Autodesk Inventor part; units mm, degrees
ref_plane "YZ Plane" through (0, 0, 0) normal (1, 0, 0) x (0, 1, 0)
ref_plane "XY Plane" through (0, 0, 0) normal (0, 0, 1) x (1, 0, 0)
sketch "Sketch1" plane through (0, 0, 0) normal (0, 1, 0) x (-1, 0, 0)
  line L0 (20, 0) -> (0, 0)
  line L1 (0, 0) -> (0, -41)
  line L2 (0, -41) -> (20, -41)
  line L3 (20, -41) -> (20, 0)
  dimension "d0" = 20
  dimension "d1" = 41
extrude "Extrusion1" add sketch "Sketch1" along normal blind 37.5
sketch "Sketch2" plane through (0, 37.5, 0) normal (0, 1, 0) x (1, 0, 0)
  circle A0 centre (-10, 31) radius 3
  line L0 (-20, 41) -> (-20, 0)
  line L1 (0, 41) -> (-20, 41)
  point P0 (0, 0)
  dimension "d4" = 6
  dimension "d5" = 10
  dimension "d6" = 10
extrude "Extrusion2" add sketch "Sketch2" along normal blind 6.5
sketch "Sketch3" plane through (0, 37.5, 0) normal (0, 1, 0) x (1, 0, 0)
  circle A0 centre (-10, 31) radius 3
  circle A1 centre (-10, 31) radius 7
  point P0 (0, 0)
  dimension "d9" = 14
extrude "Extrusion3" add sketch "Sketch3" along normal blind 2.5
chamfer "Chamfer1" distance 2.5 angle 45 1 edges at (-17, 40, -31)
ref_plane "Work Plane1" through (0, 27.5, 0) normal (0, 1, 0) x (-1, 0, 0)
sketch "Sketch4" plane through (0, 27.5, 0) normal (0, 1, 0) x (-1, 0, 0)
  line L0 (19, -47.75) -> (1, -47.75)
  line L1 (1, -47.75) -> (1, 6.75)
  line L2 (1, 6.75) -> (19, 6.75)
  line L3 (19, 6.75) -> (19, -47.75)
  line L4 (0, 0) -> (0, -41)
  line L5 (0, -41) -> (20, -41)
  line L6 (14, -44) -> (6, -44) construction
  line L7 (6, -44) -> (6, 3) construction
  line L8 (6, 3) -> (14, 3) construction
  line L9 (14, 3) -> (14, -44) construction
  circle A0 centre (14, -44) radius 2
  circle A1 centre (6, -44) radius 2
  circle A2 centre (14, 3) radius 2
  circle A3 centre (6, 3) radius 2
  dimension "d16" = 54.5
  dimension "d17" = 18
  dimension "d18" = 1
  dimension "d19" = 6.75
  dimension "d20" = 47
  dimension "d21" = 8
  dimension "d22" = 5
  dimension "d23" = 3.75
  dimension "d24" = 4
  dimension "d25" = 4
  dimension "d26" = 4
  dimension "d27" = 4
extrude "Extrusion4" add sketch "Sketch4" along normal blind 2
sketch "Sketch5" plane through (-10, 44, -31) normal (0, 1, 0) x (1, 0, 0)
  circle A0 centre (0, 0) radius 3
  circle A1 centre (0, 0) radius 1.25
  point P0 (10, -31)
  dimension "d30" = 2.5
extrude "Extrusion5" cut sketch "Sketch5" against normal blind 5 contours A1
sketch "Sketch6" plane through (0, 0, -41) normal (0, 0, -1) x (-1, 0, 0)
  line L0 (6.75, 9.5) -> (13.25, 9.5)
  line L1 (13.25, 9.5) -> (13.25, 5.5)
  line L2 (13.25, 5.5) -> (6.75, 5.5)
  line L3 (6.75, 5.5) -> (6.75, 9.5)
  line L4 (0, 0) -> (20, 0)
  line L5 (0, 0) -> (0, 37.5)
  dimension "d33" = 4
  dimension "d34" = 6.5
  dimension "d35" = 5.5
  dimension "d36" = 6.75
extrude "Extrusion6" add sketch "Sketch6" along normal blind 4.5
draft "FaceDraft1" angle 2.5 pull direction (0, 0, -1) faces at (-6.75, 8.1667, -42.5) fixed edges at (-6.75, 7.5, -45.5)
draft "FaceDraft2" angle 2.5 pull direction (0, 0, -1) faces at (-8.8512, 5.5, -42.5) fixed edges at (-10, 5.5, -45.5)
draft "FaceDraft3" angle 2.5 pull direction (0, 0, -1) faces at (-8.8512, 9.5, -42.5) fixed edges at (-10, 9.5, -45.5)
draft "FaceDraft4" angle 2.5 pull direction (0, 0, -1) faces at (-13.25, 6.8333, -42.5) fixed edges at (-13.25, 7.5, -41)
properties part number "HX-15CS_15KGs_metal_gear_servo"
The model under review builds one solid part; all positions refer to its coordinate system, in mm. A direction names the side the tool comes from. Round coordinates to 2 decimals unless told otherwise and drop trailing zeros. Order: outer loops, then holes, each group sorted by start corner. A loop starts at its lowest first (then second) coordinate and runs counter-clockwise, first axis right, second up.
(1) Mouldability with a two-part tool opening along Y and no side actions: class faces 4 (the face through (-9.9, 9.6, -43.2)), 5 (the face through (-11.25, 41.54, -31.05)), 6 (the face through (-10, 27.5, -44)), 7 (the face through (-9, 44, -30)) as released by +Y, released by -Y, zero draft, split by the parting line, or undercut.
Working result:
face 4: undercut
face 5: zero draft
face 6: undercut
face 7: released by +Y
(2) Take a section at A-A, the plane z = -44. State the section outline as (x, y) points, plus the area to 3 significant figures.
Working result:
outline: (-19, 27.5) - (-16, 27.5) - (-16, 29.5) - (-19, 29.5) - close; (-13.12, 5.43) - (-6.68, 5.43) - (-6.68, 9.57) - (-13.12, 9.57) - close; (-12, 27.5) - (-8, 27.5) - (-8, 29.5) - (-12, 29.5) - close; (-4, 27.5) - (-1, 27.5) - (-1, 29.5) - (-4, 29.5) - close
area: 46.6 mm2
(3) For P1, Ø1, axis at x = -11.5, y = 21.5, coming from the +Z side; P2, Ø5.5, axis at x = -13.5, z = 2.5, coming from the +Y side; P3, Ø5, axis at x = -6, z = 3, coming from the +Y side, all flat-tipped, find the tip position at first contact; note any pin that passes through.
Working result:
P1: stops at z = 0
P2: stops at y = 37.5
P3: stops at y = 29.5
(4) Take a section at B-B, the plane x = -18. State the section outline as (y, z) points.
Working result:
outline: (0, -41) - (27.5, -41) - (27.5, -47.75) - (29.5, -47.75) - (29.5, -41) - (37.5, -41) - (37.5, 0) - (29.5, 0) - (29.5, 6.75) - (27.5, 6.75) - (27.5, 0) - (0, 0) - close
(5) Take a section at D-D, the plane y = 25. State the section outline as (x, z) points.
Working result:
outline: (-20, -41) - (0, -41) - (0, 0) - (-20, 0) - close
(6) Tool access review of faces 1 (the face through (-10, 39, -31)), 2 (the face through (-1, 28, 3)), 3 (the face through (-10, 27.5, 3)): name each direction out of +Z, -Z, +X, -X, +Y, -Y from which nothing blocks a thin tool from reaching the whole face with its end or side.
Working result:
face 1: +Y
face 2: +Z, +X, +Y, -Y
face 3: +Z, +X, -X, -Y
(7) Wall thickness on L1, parallel to Z at x = -6, y = 29; L2, parallel to Y at x = -18.5, z = -9.5; L3, parallel to Y at x = -9.25, z = -42: over which ranges is each line inside the solid? List them lowest first.
Working result:
L1: z = -47.75 to -46, -42 to 1, 5 to 6.75
L2: y = 0 to 37.5
L3: y = 5.35 to 9.65, 27.5 to 29.5
